Geometry: final body of the model. Coordinates: model frame, mm. Round coordinates to 2 decimals unless told otherwise and drop trailing zeros. Loops run counter-clockwise (first coordinate to the right, second up) from the corner with the lowest first, then second, coordinate; pieces in that order, holes last. Notation, with made-up numbers: (13, 30.5) -> (22, 30.5) arc R18 ccw to (22, 39.5) -> close; hole circle Ø6 at (-37.75, -20.75). An arc over 180 degrees is marked (long way). Answer in a Markdown table with one row per item.
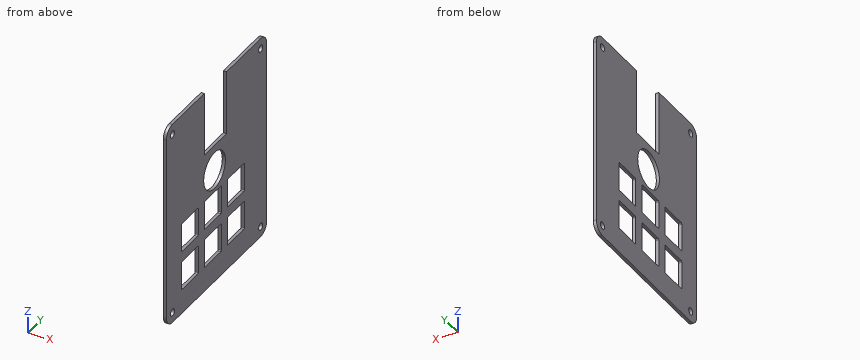
Autodesk Fusion 360 part; units mm, degrees
sketch "plate-2025-12-20T19_09_56.435Z" plane through (0, 0, 0) normal (1, 0, 0) x (0, 1, 0)
sketch "plate-2025-12-20T19_09_56.435Z (1)" plane through (0, 0, 0) normal (1, 0, 0) x (0, 1, 0)
  line L0 (18.025, 42.475) -> (31.025, 42.475)
  line L1 (18.025, 28.475) -> (31.025, 28.475)
  line L2 (17.525, 41.975) -> (17.525, 28.975)
  line L3 (31.525, 41.975) -> (31.525, 28.975)
  arc A0 (18.025, 42.475) -> (17.525, 41.975) centre (18.025, 41.975) ccw
  arc A1 (31.525, 41.975) -> (31.025, 42.475) centre (31.025, 41.975) ccw
  arc A2 (17.525, 28.975) -> (18.025, 28.475) centre (18.025, 28.975) ccw
  arc A3 (31.025, 28.475) -> (31.525, 28.975) centre (31.025, 28.975) ccw
  line L4 (37.075, 42.475) -> (50.075, 42.475)
  line L5 (37.075, 28.475) -> (50.075, 28.475)
  line L6 (36.575, 41.975) -> (36.575, 28.975)
  line L7 (50.575, 41.975) -> (50.575, 28.975)
  arc A4 (37.075, 42.475) -> (36.575, 41.975) centre (37.075, 41.975) ccw
  arc A5 (50.575, 41.975) -> (50.075, 42.475) centre (50.075, 41.975) ccw
  arc A6 (36.575, 28.975) -> (37.075, 28.475) centre (37.075, 28.975) ccw
  arc A7 (50.075, 28.475) -> (50.575, 28.975) centre (50.075, 28.975) ccw
  line L8 (56.125, 42.475) -> (69.125, 42.475)
  line L9 (56.125, 28.475) -> (69.125, 28.475)
  line L10 (55.625, 41.975) -> (55.625, 28.975)
  line L11 (69.625, 41.975) -> (69.625, 28.975)
  arc A8 (56.125, 42.475) -> (55.625, 41.975) centre (56.125, 41.975) ccw
  arc A9 (69.625, 41.975) -> (69.125, 42.475) centre (69.125, 41.975) ccw
  arc A10 (55.625, 28.975) -> (56.125, 28.475) centre (56.125, 28.975) ccw
  arc A11 (69.125, 28.475) -> (69.625, 28.975) centre (69.125, 28.975) ccw
  line L12 (18.025, 23.425) -> (31.025, 23.425)
  line L13 (18.025, 9.425) -> (31.025, 9.425)
  line L14 (17.525, 22.925) -> (17.525, 9.925)
  line L15 (31.525, 22.925) -> (31.525, 9.925)
  arc A12 (18.025, 23.425) -> (17.525, 22.925) centre (18.025, 22.925) ccw
  arc A13 (31.525, 22.925) -> (31.025, 23.425) centre (31.025, 22.925) ccw
  arc A14 (17.525, 9.925) -> (18.025, 9.425) centre (18.025, 9.925) ccw
  arc A15 (31.025, 9.425) -> (31.525, 9.925) centre (31.025, 9.925) ccw
  line L16 (37.075, 23.425) -> (50.075, 23.425)
  line L17 (37.075, 9.425) -> (50.075, 9.425)
  line L18 (36.575, 22.925) -> (36.575, 9.925)
  line L19 (50.575, 22.925) -> (50.575, 9.925)
  arc A16 (37.075, 23.425) -> (36.575, 22.925) centre (37.075, 22.925) ccw
  arc A17 (50.575, 22.925) -> (50.075, 23.425) centre (50.075, 22.925) ccw
  arc A18 (36.575, 9.925) -> (37.075, 9.425) centre (37.075, 9.925) ccw
  arc A19 (50.075, 9.425) -> (50.575, 9.925) centre (50.075, 9.925) ccw
  line L20 (56.125, 23.425) -> (69.125, 23.425)
  line L21 (56.125, 9.425) -> (69.125, 9.425)
  line L22 (55.625, 22.925) -> (55.625, 9.925)
  line L23 (69.625, 22.925) -> (69.625, 9.925)
  arc A20 (56.125, 23.425) -> (55.625, 22.925) centre (56.125, 22.925) ccw
  arc A21 (69.625, 22.925) -> (69.125, 23.425) centre (69.125, 22.925) ccw
  arc A22 (55.625, 9.925) -> (56.125, 9.425) centre (56.125, 9.925) ccw
  arc A23 (69.125, 9.425) -> (69.625, 9.925) centre (69.125, 9.925) ccw
sketch "Sketch3" plane through (0, 0, 0) normal (1, 0, 0) x (0, 1, 0)
  line L0 (5.143, 96.836) -> (88.183, 96.836)
  line L1 (88.183, 96.836) -> (88.183, -2.424)
  line L2 (88.183, -2.424) -> (5.143, -2.424)
  line L3 (5.143, -2.424) -> (5.143, 96.836)
  line L4 (18.025, 9.425) -> (31.025, 9.425)
  line L5 (17.525, 22.925) -> (17.525, 9.925)
  line L6 (36.493, 96.836) -> (54.993, 96.836)
  line L7 (54.993, 96.836) -> (54.993, 65.836)
  line L8 (54.993, 65.836) -> (36.493, 65.836)
  line L9 (36.493, 65.836) -> (36.493, 96.836)
  circle A0 centre (10.143, 2.576) radius 1.7
  circle A1 centre (83.183, 2.576) radius 1.7
  circle A2 centre (10.143, 91.836) radius 1.7
  circle A3 centre (83.183, 91.836) radius 1.7
  circle A4 centre (44.9917, 53.2578) radius 9
  dimension "d1" = 83.04
  dimension "d2" = 99.26
  dimension "d3" = 11.849
  dimension "d4" = 12.382
  dimension "d5" = 31
  dimension "d6" = 18.5
  dimension "d7" = 31.35
  dimension "d8" = 3.4
  dimension "d9" = 3.4
  dimension "d10" = 5
  dimension "d11" = 5
  dimension "d12" = 5
  dimension "d13" = 5
  dimension "d14" = 3.4
  dimension "d15" = 3.4
  dimension "d16" = 5
  dimension "d17" = 5
  dimension "d18" = 5
  dimension "d19" = 5
  dimension "d20" = 18
  dimension "d21" = 39.8487
extrude "Extrude1" add sketch "Sketch3" along normal blind 1.5 contours L0 L1 L2 L3 L7 L8 L9
extrude "Extrude2" cut sketch "plate-2025-12-20T19_09_56.435Z (1)" along normal through all
fillet "Fillet1" radius 5 1 edges at (0.75, 88.183, 96.836)
fillet "Fillet2" radius 5 1 edges at (0.75, 5.143, 96.836)
fillet "Fillet3" radius 5 1 edges at (0.75, 5.143, -2.424)
fillet "Fillet4" radius 5 1 edges at (0.75, 88.183, -2.424)
Item 1: Section query C-C, the plane y = 46.5. Output: boundary loops of the cut face in (x, z) (3 decimals), and give its area (3 significant figures).
Ans:
| item | result |
|---|---|
| outline | (0, -2.424) -> (1.5, -2.424) -> (1.5, 9.425) -> (0, 9.425) -> close; (0, 23.425) -> (1.5, 23.425) -> (1.5, 28.475) -> (0, 28.475) -> close; (0, 42.475) -> (1.5, 42.475) -> (1.5, 44.385) -> (0, 44.385) -> close; (0, 62.131) -> (1.5, 62.131) -> (1.5, 65.836) -> (0, 65.836) -> close |
| area | 33.8 mm2 |
Item 2: Ray query, L1, parallel to Z at x = 1.15, y = 57 (3 decimals); L2, parallel to Y at x = 0.45, z = 39.5 (3 decimals); L3, parallel to Y at x = 0.5, z = 80. Return the intervals inside material, ascending.
Ans:
| item | result |
|---|---|
| L1 | -2.424 to 9.425, 23.425 to 28.475, 42.475 to 96.836 |
| L2 | 5.143 to 17.525, 31.525 to 36.575, 50.575 to 55.625, 69.625 to 88.183 |
| L3 | 5.14 to 36.49, 54.99 to 88.18 |
Item 3: Section query B-B, the plane z = 78. Output: boundary loops of the cut face in (x, y), and give its area (3 significant figures).
Ans:
| item | result |
|---|---|
| outline | (0, 5.14) -> (1.5, 5.14) -> (1.5, 36.49) -> (0, 36.49) -> close; (0, 54.99) -> (1.5, 54.99) -> (1.5, 88.18) -> (0, 88.18) -> close |
| area | 96.8 mm2 |
Item 4: First-contact query: P1, Ø3, axis at y = 10.143, z = 2.576, coming from the -X side; P2, Ø23.5, axis at y = 44.99, z = 53.26, coming from the -X side. Flat tips, straight axial feed; report the tip coordinate or a pass-through.
Ans:
| item | result |
|---|---|
| P1 | through |
| P2 | x = 0 |
Item 5: Section query D-D, the plane x = 0.65. State how many separate pieces and enclosed holes the cut face has, and give its area (3 significant figures).
Ans:
| item | result |
|---|---|
| separate pieces | 1 |
| enclosed holes | 11 |
| area | 6,180 mm2 |
Item 6: Section query A-A, the plane z = 35. Output: boundary loops of the cut face in (x, y) (3 decimals).
Ans:
| item | result |
|---|---|
| outline | (0, 5.143) -> (1.5, 5.143) -> (1.5, 17.525) -> (0, 17.525) -> close; (0, 31.525) -> (1.5, 31.525) -> (1.5, 36.575) -> (0, 36.575) -> close; (0, 50.575) -> (1.5, 50.575) -> (1.5, 55.625) -> (0, 55.625) -> close; (0, 69.625) -> (1.5, 69.625) -> (1.5, 88.183) -> (0, 88.183) -> close |
